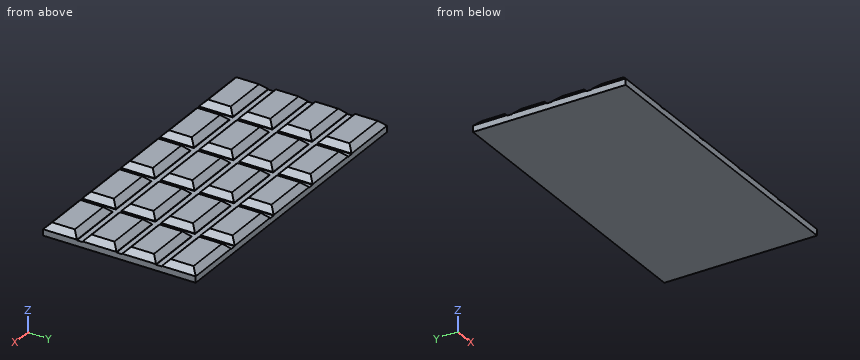
```python
from build123d import *

# Parameters (mm, degrees)
BOX001_W      = 10
BOX001_H      = 6
BOX001_DEPTH  = 1.1
CHAMFER_SIZE  = 1
ARRAY_X_COUNT = 5
ARRAY_X_PITCH = 11
ARRAY_Y_COUNT = 4
ARRAY_Y_PITCH = 7
BOX_W         = 54
BOX_H         = 27
BOX_DEPTH     = 1


with BuildPart() as obj1:
    # Box001 → Box001 (new body)
    with BuildSketch(Plane.XY.offset(1)):
        with Locations((5, 3)):
            Rectangle(BOX001_W, BOX001_H)
    extrude(amount=BOX001_DEPTH)

    # Chamfer
    chamfer_edges = [obj1.edges().sort_by_distance(p)[0] for p in [
        (0, 3, 2.1),
        (10, 3, 2.1),
        (5, 0, 2.1),
        (5, 6, 2.1),
    ]]
    chamfer(chamfer_edges, length=CHAMFER_SIZE)

    # Array X: obj1 ×5


with BuildPart() as obj1_1:
    add(obj1.part)
    with Locations(*[(i * ARRAY_X_PITCH, 0, 0) for i in range(1, ARRAY_X_COUNT)]):
        add(obj1.part)

    # Array Y: obj1 ×4


with BuildPart() as obj1_2:
    add(obj1_1.part)
    with Locations(*[(0, i * ARRAY_Y_PITCH, 0) for i in range(1, ARRAY_Y_COUNT)]):
        add(obj1_1.part)


with BuildPart() as obj2:
    # Box → Box (new body)
    with BuildSketch(Plane.XY):
        with Locations((27, 13.5)):
            Rectangle(BOX_W, BOX_H)
    extrude(amount=BOX_DEPTH)

    # Fusion: union obj1
    add(obj1_2.part)


solid = obj2.part
```
For this review, take the finished solid that the model builds, in its own axes (mm). Coordinates: 2 decimals unless noted, no trailing zeros. Write each loop counter-clockwise with the first axis right and the second up, starting at its lowest first coordinate (ties: lowest second). Pieces come first, ordered by that corner, then holes. Notation, with made-up numbers: (35, 83) - (87, 83) arc R12 ccw to (87, 97) - close; hole circle Ø9 at (-13.5, 32.5). An arc over 180 degrees is marked (long way). Put each result on its own line as item: value.
1. Wall thickness on probe 1 along X at (y, z) = (17.5, 1.05); probe 2 along Y at (x, z) = (40.5, 1.95); probe 3 along X at (y, z) = (17, 1.4): over which ranges is each line inside the solid? List them lowest first.
Values found:
probe 1: 0 to 10, 11 to 21, 22 to 32, 33 to 43, 44 to 54
probe 2: 0.85 to 5.15, 7.85 to 12.15, 14.85 to 19.15, 21.85 to 26.15
probe 3: 0.3 to 9.7, 11.3 to 20.7, 22.3 to 31.7, 33.3 to 42.7, 44.3 to 53.7
2. Add section C-C, the plane z = 1.45. Count the separate pieces of the cut face and the enclosed holes in it, then the cut area to 3 significant figures.
Values found:
separate pieces: 20
enclosed holes: 0
area: 986 mm²
3. Add section B-B, the plane x = 4. Give the boundary of the cut face in (y, z).
Values found:
outline: (0, 0) - (27, 0) - (27, 1.1) - (26, 2.1) - (22, 2.1) - (21, 1.1) - (21, 1) - (20, 1) - (20, 1.1) - (19, 2.1) - (15, 2.1) - (14, 1.1) - (14, 1) - (13, 1) - (13, 1.1) - (12, 2.1) - (8, 2.1) - (7, 1.1) - (7, 1) - (6, 1) - (6, 1.1) - (5, 2.1) - (1, 2.1) - (0, 1.1) - close
4. Add section D-D, the plane x = 22.5. Give the boundary of the cut face in (y, z), then the cut area to 3 significant figures.
Values found:
outline: (0, 0) - (27, 0) - (27, 1.1) - (26.5, 1.6) - (21.5, 1.6) - (21, 1.1) - (21, 1) - (20, 1) - (20, 1.1) - (19.5, 1.6) - (14.5, 1.6) - (14, 1.1) - (14, 1) - (13, 1) - (13, 1.1) - (12.5, 1.6) - (7.5, 1.6) - (7, 1.1) - (7, 1) - (6, 1) - (6, 1.1) - (5.5, 1.6) - (0.5, 1.6) - (0, 1.1) - close
area: 40.4 mm²
5. For pin 1 (4 mm diameter, centred on x = 48, y = 21.5, fed in from +Z), flat-tipped, find the tip position at first contact; note if it passes through.
Values found:
pin 1: z = 2.1
